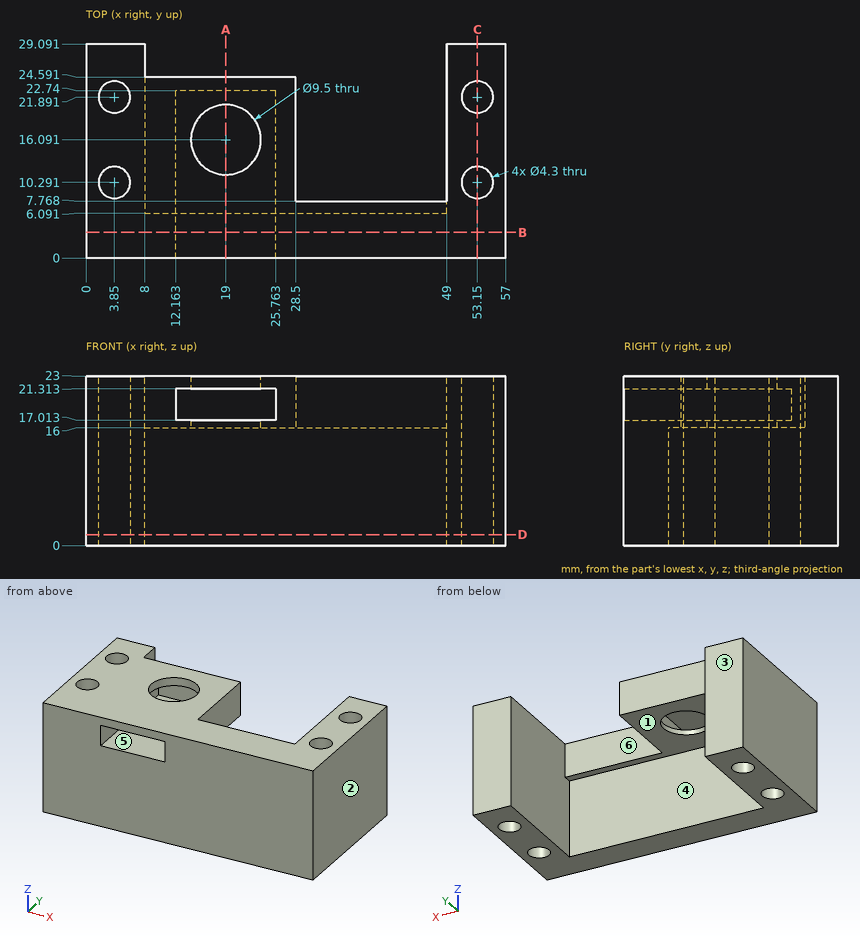
The figure shows three views and two pictorial views of one solid part (mm, origin at its lowest corner). Answer the questions. A direction names the side the tool comes from. Coordinates: 2 decimals unless noted, no trailing zeros. Loops run counter-clockwise (first coordinate to the right, second up) from the corner with the lowest first, then second, coordinate; pieces in that order, holes last. Notation, with made-up numbers: (-27, 55.5) -> (-11, 55.5) arc R23 ccw to (-11, 89.5) -> close; hole circle Ø8 at (-16.75, 50.25). An arc over 180 degrees is marked (long way). Return JSON: item names as keys, results as strings. Group by question number.
(1) A cutting plane is placed at D-D on z = 1.5. Write down the section's boundary in (x, y).
(2) Given pin 1 Ø2 at (x, z) = (42.5, 2.5) entering from +Y; pin 2 Ø2.5 at (x, y) = (53.15, 21.89) entering from +Z; pin 3 Ø11 at (x, y) = (19, 16.09) entering from -Z, each flat-ended and moving along its own axis, determine where each tip first touches the part or whether it passes through.
(3) A cutting plane is placed at C-C on x = 53.15. Write down the section's boundary in (y, z).
(4) A cutting plane is placed at A-A on x = 19. Write down the section's boundary in (y, z).
(5) Which of the six approach directions +Z, -Z, +X, -X, +Y, -Y give full straight-line access (tool end or side, diameter ignored) to the marked faces 4, 5 and 6?
(6) Find the intervals of material crossed by probe 1 along Y at (x, z) = (3.85, 13.75); probe 2 along X at (y, z) = (8.75, 7.25); probe 3 along Y at (x, z) = (3, 1.25), in increasing order. Write a range as from..to.
(7) A cutting plane is placed at B-B on y = 3.5. Write down the section's boundary in (x, z), and give its area (3 significant figures).
(8) Determine the mould class of the marked faces 1, 2 and 3 for opening direction X: released by +X, released by -X, zero draft, split by the parting line, or undercut.
The answers:
{
 "1": {"outline": "(0, 0) -> (57, 0) -> (57, 29.09) -> (49, 29.09) -> (49, 6.09) -> (8, 6.09) -> (8, 29.09) -> (0, 29.09) -> close; hole circle Ø4.3 at (3.85, 10.29); hole circle Ø4.3 at (3.85, 21.89); hole circle Ø4.3 at (53.15, 10.29); hole circle Ø4.3 at (53.15, 21.89)"},
 "2": {"pin 1": "stops at y = 6.09", "pin 2": "passes through", "pin 3": "stops at z = 16"},
 "3": {"outline": "(0, 0) -> (8.14, 0) -> (8.14, 23) -> (0, 23) -> close; (12.44, 0) -> (19.74, 0) -> (19.74, 23) -> (12.44, 23) -> close; (24.04, 0) -> (29.09, 0) -> (29.09, 23) -> (24.04, 23) -> close"},
 "4": {"outline": "(0, 0) -> (6.09, 0) -> (6.09, 16) -> (11.34, 16) -> (11.34, 17.01) -> (0, 17.01) -> close; (0, 21.31) -> (11.34, 21.31) -> (11.34, 23) -> (0, 23) -> close; (20.84, 16) -> (24.59, 16) -> (24.59, 23) -> (20.84, 23) -> (20.84, 21.31) -> (22.74, 21.31) -> (22.74, 17.01) -> (20.84, 17.01) -> close"},
 "5": {"face 4": "-Z, +Y", "face 5": "-Y", "face 6": "+Z, -Z, +Y"},
 "6": {"probe 1": "y = 0..8.14, 12.44..19.74, 24.04..29.09", "probe 2": "x = 0..2.35, 5.35..8, 49..51.65, 54.65..57", "probe 3": "y = 0..8.32, 12.27..19.92, 23.87..29.09"},
 "7": {"outline": "(0, 0) -> (57, 0) -> (57, 23) -> (0, 23) -> close; hole (12.16, 17.01) -> (25.76, 17.01) -> (25.76, 21.31) -> (12.16, 21.31) -> close", "area": "1,250 mm^2"},
 "8": {"face 1": "undercut", "face 2": "released by +X", "face 3": "zero draft"}
}
